Geometry check sheet. Reference: the model listing, model coordinates, mm. A direction names the side the tool comes from. Round coordinates to 2 decimals unless told otherwise and drop trailing zeros. Order: outer loops, then holes, each group sorted by start corner. A loop starts at its lowest first (then second) coordinate and runs counter-clockwise, first axis right, second up. Notation, with made-up numbers: (58.25, 65) - (72.25, 65) arc R24 cw to (72.25, 104) - close; hole circle Ø4 at (-3.75, 77.25). An arc over 180 degrees is marked (long way). One line per question, with ' | ' between items. Start each with the question number.
Q1. Sectioned sample at B-B, the plane z = 18.5. Enter the section's corners in (x, y) (1 decimal).
Q2. Sectioned sample at C-C, the plane y = -9.75. Enter the section's corners in (x, z) (3 decimals).
Q3. Sectioned sample at D-D, the plane z = 27.5. Enter the section's corners in (x, y).
Q4. Material ranges on line 1 along Y through (x, z) = (6, 18.5); line 2 along X through (y, z) = (0.25, 19); line 3 along X through (y, z) = (7, 5), recorded low to high.
Q5. Tool access check on faces 1 (the face through (-11, 3.969, 8)), 2 (the face through (-2.5, -12.93, 11.83)), 3 (the face through (11, -3.969, 12)), 4 (the face through (2.85, 4.77, 8.01)). Record the directions out of +Z, -Z, +X, -X, +Y, -Y that give a thin tool (end or side, any length) a straight path to the whole face; none if there is none.
Q6. Sectioned sample at A-A, the plane x = 0. Enter the section's corners in (y, z) (1 decimal), then the cut area to 3 significant figures.
Q7. Gauge pin test, flat ends, axial feed: P1, Ø1, axis at x = -5.5, z = 8, coming from the -Y side; P2, Ø6, axis at x = 0.5, y = 8, coming from the -Z side; P3, Ø1.8, axis at x = 10.5, z = 14, coming from the +Y side; P4, Ø4.5, axis at x = 7, y = -11, coming from the -Z side. Record the tip position at first contact, or that the pin passes through.
Q8. Mould release check, pull along Y, two halves, no side actions. Record for faces 5 (the face through (-7, -9, 4.445)), 6 (the face through (0, -3.437, 42)), 7 (the face through (7, 10, 16.243)), 8 (the face through (3, 2, 40.958)): +Y half, -Y half, draft (parallel to the pull), parting line (faces both ways), or undercut.
```python
from build123d import *

# Parameters (mm, degrees)
F0_R      = 13.49375
F0_R_2    = 2.15265
F1_DEPTH  = 19.4183
F5_DEPTH  = 14.9733
F7_DEPTH  = 16.2433
F8_R      = 5.55625
F8_R_2    = 2.15265
F9_DEPTH  = 12.6492
F10_R     = 3.96875
F10_R_2   = 2.15265
F11_DEPTH = 8.89
F12_R     = 2.15265
F13_DEPTH = 1.5875
F14_R     = 0.762


with BuildPart() as f1:
    # F0 (on Top) → F1 (new body)
    with BuildSketch(Plane.XY):
        Circle(F0_R)
        with Locations((-4.7625, -8.248892)):
            Circle(F0_R_2, mode=Mode.SUBTRACT)
        with Locations((4.7625, -8.248892)):
            Circle(F0_R_2, mode=Mode.SUBTRACT)
        with Locations((-9.525, 0)):
            Circle(F0_R_2, mode=Mode.SUBTRACT)
        with Locations((-4.7625, 8.248892)):
            Circle(F0_R_2, mode=Mode.SUBTRACT)
        Circle(F0_R_2, mode=Mode.SUBTRACT)
        with Locations((9.525, 0)):
            Circle(F0_R_2, mode=Mode.SUBTRACT)
        with Locations((4.7625, 8.248892)):
            Circle(F0_R_2, mode=Mode.SUBTRACT)
    extrude(amount=F1_DEPTH)

    # F4 (on face) → F5 (cut, through all)
    with BuildSketch(Plane.XY.offset(19.4183)):
        with BuildLine():
            Line((-3.309837, 13.670305), (-10.183913, 9.701555))
            Line((-10.183913, 9.701555), (-8.199538, 6.264517))
            ThreePointArc((-8.199538, 6.264517), (-2.778125, 4.811854), (-1.325462, 10.233267))
            Line((-1.325462, 10.233267), (-3.309837, 13.670305))
        make_face()
        with BuildLine():
            Line((13.49375, 3.96875), (9.525, 3.96875))
            ThreePointArc((9.525, 3.96875), (5.55625, 0), (9.525, -3.96875))
            Line((9.525, -3.96875), (13.49375, -3.96875))
            Line((13.49375, -3.96875), (13.49375, 3.96875))
        make_face()
        with BuildLine():
            Line((-8.199538, -6.264517), (-10.183913, -9.701555))
            Line((-10.183913, -9.701555), (-3.309837, -13.670305))
            Line((-3.309837, -13.670305), (-1.325462, -10.233267))
            ThreePointArc((-1.325462, -10.233267), (-2.778125, -4.811854), (-8.199538, -6.264517))
        make_face()
    extrude(amount=-F5_DEPTH, mode=Mode.SUBTRACT)

    # F6 (on face) → F7 (cut, through all)
    with BuildSketch(Plane(origin=(0, 0, 0), x_dir=(1, 0, 0), z_dir=(0, 0, -1))):
        with BuildLine():
            Line((1.325462, -10.233267), (3.309837, -13.670305))
            Line((3.309837, -13.670305), (10.183913, -9.701555))
            Line((10.183913, -9.701555), (8.199538, -6.264517))
            ThreePointArc((8.199538, -6.264517), (2.778125, -4.811854), (1.325462, -10.233267))
        make_face()
        with BuildLine():
            Line((10.183913, 9.701555), (3.309837, 13.670305))
            Line((3.309837, 13.670305), (1.325462, 10.233267))
            ThreePointArc((1.325462, 10.233267), (2.778125, 4.811854), (8.199538, 6.264517))
            Line((8.199538, 6.264517), (10.183913, 9.701555))
        make_face()
        with BuildLine():
            Line((-9.525, 3.96875), (-13.49375, 3.96875))
            Line((-13.49375, 3.96875), (-13.49375, -3.96875))
            Line((-13.49375, -3.96875), (-9.525, -3.96875))
            ThreePointArc((-9.525, -3.96875), (-5.55625, 0), (-9.525, 3.96875))
        make_face()
    extrude(amount=-F7_DEPTH, mode=Mode.SUBTRACT)

    # F8 (on face) → F9 (join)
    with BuildSketch(Plane.XY.offset(19.4183)):
        Circle(F8_R)
        Circle(F8_R_2, mode=Mode.SUBTRACT)
    extrude(amount=F9_DEPTH)

    # F10 (on face) → F11 (join)
    with BuildSketch(Plane.XY.offset(32.0675)):
        Circle(F10_R)
        Circle(F10_R_2, mode=Mode.SUBTRACT)
    extrude(amount=F11_DEPTH)

    # F12 (on face) → F13 (join)
    with BuildSketch(Plane.XY.offset(40.9575)):
        Polygon((1.984375, 3.437038), (-1.984375, 3.437038), (-3.96875, 0), (-1.984375, -3.437038), (1.984375, -3.437038), (3.96875, 0), align=None)
        Circle(F12_R, mode=Mode.SUBTRACT)
    extrude(amount=F13_DEPTH)

    # F14
    f14_edges = [f1.edges().sort_by_distance(p)[0] for p in [
        (-9.885494, -9.184678, 11.93165),
        (3.011417, -13.153428, 8.12165),
        (9.885494, -9.184678, 8.12165),
        (12.896911, 3.96875, 11.93165),
        (12.896911, -3.96875, 11.93165),
        (-3.011417, -13.153428, 11.93165),
        (9.885494, 9.184678, 8.12165),
        (3.011417, 13.153428, 8.12165),
        (-3.011417, 13.153428, 11.93165),
        (-9.885494, 9.184678, 11.93165),
        (-12.896911, 3.96875, 8.12165),
        (-12.896911, -3.96875, 8.12165),
    ]]
    fillet(f14_edges, radius=F14_R)


solid = f1.part
```
Determined:
1) outline: (-10.6, -8.3) arc R0.8 ccw to (-9.3, -8.3) - (-8.2, -6.3) arc R4 cw to (-1.3, -10.2) - (-2.5, -12.2) arc R0.8 ccw to (-1.9, -13.4) arc R13.5 ccw to (12.5, -5) arc R0.8 ccw to (11.8, -4) - (9.5, -4) arc R4 cw to (9.5, 4) - (11.8, 4) arc R0.8 ccw to (12.5, 5) arc R13.5 ccw to (-1.9, 13.4) arc R0.8 ccw to (-2.5, 12.2) - (-1.3, 10.2) arc R4 cw to (-8.2, 6.3) - (-9.3, 8.3) arc R0.8 ccw to (-10.6, 8.3) arc R13.5 ccw to start; hole circle Ø4.3 at (-9.5, 0); hole circle Ø4.3 at (0, 0); hole circle Ø4.3 at (4.8, -8.2); hole circle Ø4.3 at (4.8, 8.2)
2) outline: (-9.328, 0) - (-6.305, 0) - (-6.305, 4.445) - (-9.328, 4.445) - close; (-3.22, 0) - (1.089, 0) - (1.089, 16.243) - (3.22, 16.243) - (3.22, 19.418) - (-1.089, 19.418) - (-1.089, 4.445) - (-3.22, 4.445) - close; (6.305, 16.243) - (9.328, 16.243) - (9.328, 19.418) - (6.305, 19.418) - close
3) outline: circle Ø11.11 at (0, 0); hole circle Ø4.31 at (0, 0)
4) line 1: y = -12.09 to -10.01, -6.49 to -1.82, 1.82 to 6.49, 10.01 to 12.09 | line 2: x = -13.49 to -11.66, -7.39 to -2.14, 2.14 to 5.56 | line 3: x = -11.54 to -8.62, -1 to 1, 8.62 to 11.54
5) face 1: -Z, -X | face 2: +Z, -X | face 3: +Z, +X | face 4: -Z
6) outline: (-13.5, 0) - (-2.2, 0) - (-2.2, 42.5) - (-3.4, 42.5) - (-3.4, 41) - (-4, 41) - (-4, 32.1) - (-5.6, 32.1) - (-5.6, 19.4) - (-13.5, 19.4) - close; (2.2, 0) - (13.5, 0) - (13.5, 19.4) - (5.6, 19.4) - (5.6, 32.1) - (4, 32.1) - (4, 41) - (3.4, 41) - (3.4, 42.5) - (2.2, 42.5) - close | area: 563 mm2
7) P1: stops at y = -4.48 | P2: stops at z = 0 | P3: stops at y = 8.63 | P4: stops at z = 16.24
8) face 5: undercut | face 6: -Y half | face 7: undercut | face 8: draft
